from build123d import *

# Parameters (mm, degrees)
SKETCH1_W            = 24
SKETCH1_H            = 15
BOSS_EXTRUDE1_DEPTH  = 0.75
BOSS_EXTRUDE2_START  = -1.5
BOSS_EXTRUDE2_DEPTH  = 4
MIRROR2_START        = -1.5
MIRROR2_COPY_1_DEPTH = 4
SKETCH3_R            = 1.2
BOSS_EXTRUDE3_DEPTH  = 1.5
FILLET1_R            = 1
BOSS_EXTRUDE4_DEPTH  = 1.5
SKETCH5_W            = 12.692307692
SKETCH5_H            = 7.5
CUT_EXTRUDE1_DEPTH   = 1.5
FILLET2_R            = 1.5


with BuildPart() as part:
    # Sketch1 → Boss-Extrude1 (new, symmetric)
    with BuildSketch(Plane(origin=(0, 0, 0), x_dir=(1, 0, 0), z_dir=(0, 1, 0))):
        Rectangle(SKETCH1_W, SKETCH1_H)
    extrude(amount=BOSS_EXTRUDE1_DEPTH, both=True)

    # Sketch2 → Boss-Extrude2 (add)
    with BuildSketch(Plane(origin=(0, 0.75, 0), x_dir=(1, 0, 0), z_dir=(0, 1, 0)).offset(BOSS_EXTRUDE2_START)):
        Polygon((-12, 4.5), (-14, 4.5), (-14, 9.5), (-9, 9.5), (-9, 7.5), (-12, 7.5), align=None)
    boss_extrude2 = extrude(amount=BOSS_EXTRUDE2_DEPTH)

    # Mirror1: Boss-Extrude2 across plane
    add(boss_extrude2.mirror(Plane(origin=(0, 0, 0), x_dir=(0, 0, 1), z_dir=(1, 0, 0))))

    # Mirror2: Boss-Extrude2 across plane
    add(boss_extrude2.mirror(Plane.XY))

    # Mirror2 copy 1 sketch → Mirror2 copy 1 (add)
    with BuildSketch(Plane(origin=(0, 0.75, 0), x_dir=(-1, 0, 0), z_dir=(0, 1, 0)).offset(MIRROR2_START)):
        Polygon((-12, 4.5), (-14, 4.5), (-14, 9.5), (-9, 9.5), (-9, 7.5), (-12, 7.5), align=None)
    extrude(amount=MIRROR2_COPY_1_DEPTH)

    # Sketch3 → Boss-Extrude3 (add)
    # profile 1 of 4: a face of its own
    with BuildSketch(Plane(origin=(0, 0.75, 0), x_dir=(1, 0, 0), z_dir=(0, 1, 0))):
        with BuildLine():
            Line((-17.67766953, 2.7), (-12, 2.7))
            Line((-12, 2.7), (-12, -2.7))
            Line((-12, -2.7), (-17.67766953, -2.7))
            ThreePointArc((-17.67766953, -2.7), (-20.37766953, 0), (-17.67766953, 2.7))
        make_face()
        with Locations(Location((-17.67766953, 0, 0), (0, 0, 270))):
            Circle(SKETCH3_R, mode=Mode.SUBTRACT)
    # profile 2 of 4: a face of its own
    with BuildSketch(Plane(origin=(0, 0.75, 0), x_dir=(1, 0, 0), z_dir=(0, 1, 0))):
        with BuildLine():
            Line((-2.7, 17.67766953), (-2.7, 7.5))
            Line((-2.7, 7.5), (2.7, 7.5))
            Line((2.7, 7.5), (2.7, 17.67766953))
            ThreePointArc((2.7, 17.67766953), (0, 20.37766953), (-2.7, 17.67766953))
        make_face()
        with Locations(Location((0, 17.67766953, 0), (0, 0, 270))):
            Circle(SKETCH3_R, mode=Mode.SUBTRACT)
    # profile 3 of 4: a face of its own
    with BuildSketch(Plane(origin=(0, 0.75, 0), x_dir=(1, 0, 0), z_dir=(0, 1, 0))):
        with BuildLine():
            Line((12, -2.7), (17.67766953, -2.7))
            ThreePointArc((17.67766953, -2.7), (20.37766953, 0), (17.67766953, 2.7))
            Line((17.67766953, 2.7), (12, 2.7))
            Line((12, 2.7), (12, -2.7))
        make_face()
        with Locations(Location((17.67766953, 0, 0), (0, 0, 90))):
            Circle(SKETCH3_R, mode=Mode.SUBTRACT)
    # profile 4 of 4: a face of its own
    with BuildSketch(Plane(origin=(0, 0.75, 0), x_dir=(1, 0, 0), z_dir=(0, 1, 0))):
        with BuildLine():
            Line((-2.7, -7.5), (2.7, -7.5))
            Line((2.7, -7.5), (2.7, -17.67766953))
            ThreePointArc((2.7, -17.67766953), (0, -20.37766953), (-2.7, -17.67766953))
            Line((-2.7, -17.67766953), (-2.7, -7.5))
        make_face()
        with Locations(Location((0, -17.67766953, 0), (0, 0, 90))):
            Circle(SKETCH3_R, mode=Mode.SUBTRACT)
    extrude(amount=-BOSS_EXTRUDE3_DEPTH)

    # Fillet1
    fillet1_edges = [part.edges().sort_by_distance(p)[0] for p in [
        (-14, 1.25, 9.5),
        (-14, 3.25, 7),
        (-11.5, 3.25, 9.5),
        (14, 1.25, 9.5),
        (11.5, 3.25, 9.5),
        (14, 3.25, 7),
        (14, 1.25, -9.5),
        (14, 3.25, -7),
        (11.5, 3.25, -9.5),
        (-11.5, 3.25, -9.5),
        (-14, 3.25, -7),
        (-14, 1.25, -9.5),
        (-10.5, 0.75, -7.5),
        (-12, 0.75, -6),
        (10.5, 0.75, -7.5),
        (12, 0.75, -6),
        (12, 0.75, 6),
        (10.5, 0.75, 7.5),
        (-10.5, 0.75, 7.5),
        (-12, 0.75, 6),
        (2.7, 0, -7.5),
        (-2.7, 0, -7.5),
        (-2.7, 0, 7.5),
        (2.7, 0, 7.5),
        (12, 0, 2.7),
        (12, 0, -2.7),
        (-12, 0, 2.7),
        (-12, 0, -2.7),
    ]]
    fillet(fillet1_edges, radius=FILLET1_R)

    # Sketch4 → Boss-Extrude4 (add)
    with BuildSketch(Plane(origin=(0, 0.75, 0), x_dir=(1, 0, 0), z_dir=(0, 1, 0))):
        with BuildLine():
            Line((-12.8, -4.5), (-12, -4.5))
            Line((-12, -4.5), (-12, -3.7))
            ThreePointArc((-12, -3.7), (-12.234314575, -4.265685425), (-12.8, -4.5))
        make_face()
        with BuildLine():
            Line((-12.8, 4.5), (-12, 4.5))
            Line((-12, 4.5), (-12, 3.7))
            ThreePointArc((-12, 3.7), (-12.234314575, 4.265685425), (-12.8, 4.5))
        make_face()
        with BuildLine():
            Line((12.8, 4.5), (12, 4.5))
            Line((12, 4.5), (12, 3.7))
            ThreePointArc((12, 3.7), (12.234314575, 4.265685425), (12.8, 4.5))
        make_face()
        with BuildLine():
            Line((12, -3.7), (12, -4.5))
            Line((12, -4.5), (12.8, -4.5))
            ThreePointArc((12.8, -4.5), (12.234314575, -4.265685425), (12, -3.7))
        make_face()
        with BuildLine():
            Line((-9, 8.5), (-9, 7.5))
            Line((-9, 7.5), (-8, 7.5))
            ThreePointArc((-8, 7.5), (-8.707106781, 7.792893219), (-9, 8.5))
        make_face()
        with BuildLine():
            Line((8, 7.5), (9, 7.5))
            Line((9, 7.5), (9, 8.5))
            ThreePointArc((9, 8.5), (8.707106781, 7.792893219), (8, 7.5))
        make_face()
        with BuildLine():
            Line((8, -7.5), (9, -7.5))
            Line((9, -7.5), (9, -8.5))
            ThreePointArc((9, -8.5), (8.707106781, -7.792893219), (8, -7.5))
        make_face()
        with BuildLine():
            Line((-9, -8.5), (-9, -7.5))
            Line((-9, -7.5), (-8, -7.5))
            ThreePointArc((-8, -7.5), (-8.707106781, -7.792893219), (-9, -8.5))
        make_face()
    extrude(amount=-BOSS_EXTRUDE4_DEPTH)

    # Sketch5 → Cut-Extrude1 (cut)
    with BuildSketch(Plane(origin=(0, 0.75, 0), x_dir=(1, 0, 0), z_dir=(0, 1, 0))):
        Rectangle(SKETCH5_W, SKETCH5_H)
    extrude(amount=-CUT_EXTRUDE1_DEPTH, mode=Mode.SUBTRACT)

    # Fillet2
    fillet2_edges = [part.edges().sort_by_distance(p)[0] for p in [
        (6.346153846, 0, 3.75),
        (6.346153846, 0, -3.75),
        (-6.346153846, 0, -3.75),
        (-6.346153846, 0, 3.75),
    ]]
    fillet(fillet2_edges, radius=FILLET2_R)


solid = part.part
Could you check a few things on this model? Use its own coordinates, in mm. A direction names the side the tool comes from. Round coordinates to 2 decimals unless told otherwise and drop trailing zeros. Loops run counter-clockwise (first coordinate to the right, second up) from the corner with the lowest first, then second, coordinate; pieces in that order, holes last. Notation, with made-up numbers: (52, 21) -> (56, 21) arc R29 cw to (56, 43) -> close; hole circle Ø4 at (-3.75, 26). An arc over 180 degrees is marked (long way). Use CSV: the item, a comma, the result in double quotes.
(1) Suppose I cut it at D-D on x = -7.5. Write out the boundary of the cut face in (y, z), plus the area to 3 significant figures.
Return value:
outline,"(-0.75, -7.5) -> (0.75, -7.5) -> (0.75, 7.5) -> (-0.75, 7.5) -> close"
area,"22.5 mm²"
(2) For faces 1 (the cylindrical face through (5.92, -0.01, -3.3)), 2 (the cylindrical face through (11.699, 1.035, -6.021)), 3 (the flat face through (14, 1, -6)), 4 (the flat face through (9, 1, 8)), 5 (the flat face through (-13, 1, -4.5)), which set-ups out of +Z, -Z, +X, -X, +Y, -Y let a thin tool reach every point of the face, with its end or its side?
Return value:
face 1,"+Y, -Y"
face 2,"+Y"
face 3,"-Z, +X, +Y, -Y"
face 4,"+Z, +Y"
face 5,"-X, +Y"
(3) Suppose I cut it at A-A on x = 0. Write out the boundary of the cut face in (y, z).
Return value:
outline,"(-0.75, -20.38) -> (0.75, -20.38) -> (0.75, -18.88) -> (-0.75, -18.88) -> close; (-0.75, -16.48) -> (0.75, -16.48) -> (0.75, -3.75) -> (-0.75, -3.75) -> close; (-0.75, 3.75) -> (0.75, 3.75) -> (0.75, 16.48) -> (-0.75, 16.48) -> close; (-0.75, 18.88) -> (0.75, 18.88) -> (0.75, 20.38) -> (-0.75, 20.38) -> close"
(4) If we mould it in two halves opening along X, with no side actions, what happens to faces 6 (the cylindrical face through (-3.001, -0.01, -7.785)), 7 (the cylindrical face through (-12.285, -0.01, -3.001)), 8 (the flat face through (13, 1, 4.5))? For each: +X half, -X half, draft (parallel to the pull), parting line (faces both ways), or undercut.
Return value:
face 6,"undercut"
face 7,"-X half"
face 8,"draft"
(5) Will these pins go through, and if not, where does the flat tip stop? pin 1 Ø1.2 at (y, z) = (2, 5.5) entering from -X; pin 2 Ø0.5 at (x, y) = (-11, 2.5) entering from -Z; pin 3 Ø2 at (y, z) = (0, -13) entering from +X.
Return value:
pin 1,"stops at x = -14"
pin 2,"stops at z = -9.5"
pin 3,"stops at x = 2.7"
(6) Suppose I cut it at C-C on z = -7. Write out the boundary of the cut face in (x, y).
Return value:
outline,"(-14, -0.75) -> (14, -0.75) -> (14, 2.25) arc R1 ccw to (13, 3.25) -> (12, 3.25) -> (12, 1.75) arc R1 cw to (11.5, 0.88) -> (9, 0.88) -> (9, 0.75) -> (-9, 0.75) -> (-9, 0.88) -> (-11.5, 0.88) arc R1 cw to (-12, 1.75) -> (-12, 3.25) -> (-13, 3.25) arc R1 ccw to (-14, 2.25) -> close"
(7) Suppose I cut it at B-B on z = 0. Write out the boundary of the cut face in (x, y), plus the area to 3 significant figures.
Return value:
outline,"(-20.38, -0.75) -> (-18.88, -0.75) -> (-18.88, 0.75) -> (-20.38, 0.75) -> close; (-16.48, -0.75) -> (-6.35, -0.75) -> (-6.35, 0.75) -> (-16.48, 0.75) -> close; (6.35, -0.75) -> (16.48, -0.75) -> (16.48, 0.75) -> (6.35, 0.75) -> close; (18.88, -0.75) -> (20.38, -0.75) -> (20.38, 0.75) -> (18.88, 0.75) -> close"
area,"34.9 mm²"
(8) If I drill on probe 1 along X at (y, z) = (-0.15, 0); probe 2 along Z at (x, y) = (4.5, 0.6); probe 3 along Y at (x, z) = (6.5, 6), over which ranges is the centre line in solid material (lowest first)? Write a range as [from, to].
Return value:
probe 1,"x = [-20.38, -18.88], [-16.48, -6.35], [6.35, 16.48], [18.88, 20.38]"
probe 2,"z = [-7.5, -3.75], [3.75, 7.5]"
probe 3,"y = [-0.75, 0.75]"
